from build123d import *

# Parameters (mm, degrees)
F0_W     = 431.8
F0_H     = 381
F1_DEPTH = 228.6
F2_T     = 12.7


with BuildPart() as f1:
    # F0 (on Front) → F1 (new body)
    with BuildSketch(Plane.XZ):
        Rectangle(F0_W, F0_H)
    extrude(amount=F1_DEPTH)

    # F2
    f2_openings = [f1.faces().sort_by_distance(p)[0] for p in [
        (0, -114.3, 190.5),
    ]]
    offset(amount=F2_T, openings=f2_openings, kind=Kind.INTERSECTION)


solid = f1.part
Here's how the part is built. I have some questions about the finished solid (model axes, mm). A direction names the side the tool comes from. Round coordinates to 2 decimals unless told otherwise and drop trailing zeros. Order: outer loops, then holes, each group sorted by start corner. A loop starts at its lowest first (then second) coordinate and runs counter-clockwise, first axis right, second up. Notation, with made-up numbers: M -3,64 L 8,64 A18 cw 8,69 Z; hole C -26,72.5 d6. An arc over 180 degrees is marked long. Return JSON: item names as keys, results as strings. Group by question number.
1. If we section it at B-B on y = -39: List the corners of the cut face in (x, z) for me, then the cut area to 3 significant figures.
2. Please list where these lines run through material, in increasing order: probe 1 along Y at (x, z) = (86.5, 168.5); probe 2 along X at (y, z) = (-122, -100.5); probe 3 along Z at (x, y) = (63, -151.5).
3. If we section it at C-C on x = 147: List the corners of the cut face in (y, z) for me, then the cut area to 3 significant figures.
4. I'm going to push a flat-ended pin straight in: pin 1 Ø3 at (x, y) = (-144.5, -68.5) entering from +Z. Where does the tip first touch, or does it pass through?
5. If we section it at A-A on z = -26: List the corners of the cut face in (x, y) for me, then the cut area to 3 significant figures.
6. On a 3-axis mill with a long thin cutter (end or side, diameter ignored), from which of +Z, -Z, +X, -X, +Y, -Y can I reach the whole of each face in a straight line? I mean faces 1 (the face through (-3, -113, -190.5)), 2 (the face through (-228.6, -113, -9)). Say none if no direction works.
7. If we mould it in two halves opening along Y, with no side actions, what happens to faces 3 (the face through (-215.9, -113, -3)), 4 (the face through (-3, 12.7, -4)), 5 (the face through (-3, -241.3, -4))? For each: pulls with the +Y half, pulls with the -Y half, needs draft (parallel to the pull), parting line crosses it, or undercut.
Reply:
{
 "1": {"outline": "M -228.6,-203.2 L 228.6,-203.2 L 228.6,190.5 L 215.9,190.5 L 215.9,-190.5 L -215.9,-190.5 L -215.9,190.5 L -228.6,190.5 Z", "area": "15,500 mm^2"},
 "2": {"probe 1": "-241.3 to -228.6, 0 to 12.7", "probe 2": "-228.6 to -215.9, 215.9 to 228.6", "probe 3": "-203.2 to -190.5"},
 "3": {"outline": "M -241.3,-203.2 L 12.7,-203.2 L 12.7,190.5 L 0,190.5 L 0,-190.5 L -228.6,-190.5 L -228.6,190.5 L -241.3,190.5 Z", "area": "12,900 mm^2"},
 "4": {"pin 1": "z = -190.5"},
 "5": {"outline": "M -228.6,-241.3 L 228.6,-241.3 L 228.6,12.7 L -228.6,12.7 Z; hole M -215.9,-228.6 L 215.9,-228.6 L 215.9,0 L -215.9,0 Z", "area": "17,400 mm^2"},
 "6": {"face 1": "+Z", "face 2": "+Z, -Z, -X, +Y, -Y"},
 "7": {"face 3": "undercut", "face 4": "pulls with the +Y half", "face 5": "pulls with the -Y half"}
}
